Part model, mm, in its own coordinate system. Face numbers are marked on the shaded views. Give positions to 0.01 mm unless a question says otherwise; leave off trailing zeros. Write each loop counter-clockwise with the first axis right and the second up, starting at its lowest first coordinate (ties: lowest second). Pieces come first, ordered by that corner, then holes.
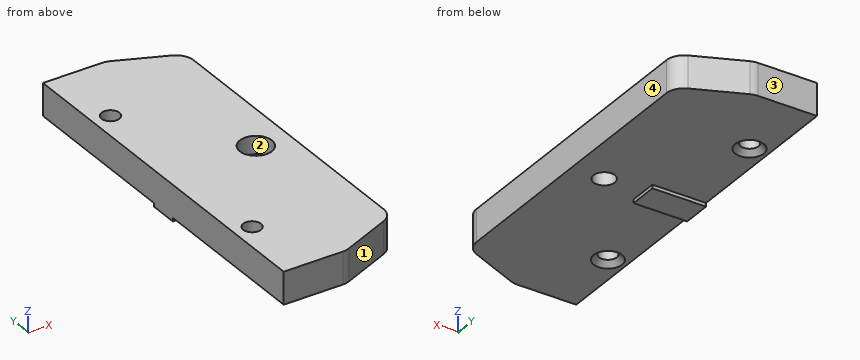
from build123d import *

# Parameters (mm, degrees)
F0_W           = 30
F0_H           = 16
F1_DEPTH       = 18
F2_D           = 12
F2_CBORE_D     = 18
F2_CBORE_DEPTH = 10
F3_DEPTH       = 20
F4_D           = 10
F4_CSINK_D     = 16
F4_CSINK_ANGLE = 90


with BuildPart() as f1:
    # F0 (on Top) → F1 (new body)
    with BuildSketch(Plane.XY):
        with BuildLine():
            Line((33.001347, 0), (0, 0))
            Line((0, 0), (0, -94))
            Line((0, -94), (30, -94))
            Line((30, -94), (30, -110))
            Line((30, -110), (0, -110))
            Line((0, -110), (0, -204))
            Line((0, -204), (33.001347, -204))
            ThreePointArc((33.001347, -204), (35.014898, -203.795183), (36.945967, -203.189123))
            Line((36.945967, -203.189123), (63.94462, -191.599396))
            ThreePointArc((63.94462, -191.599396), (68.350036, -187.912719), (70, -182.410274))
            Line((70, -182.410274), (70, -21.589726))
            ThreePointArc((70, -21.589726), (68.350036, -16.087281), (63.94462, -12.400604))
            Line((63.94462, -12.400604), (36.945967, -0.810877))
            ThreePointArc((36.945967, -0.810877), (35.014898, -0.204817), (33.001347, 0))
        make_face()
        with Locations((15, -102)):
            Rectangle(F0_W, F0_H)
    extrude(amount=-F1_DEPTH)

    # F2 (through all)
    with Locations(Plane.XY):
        with Locations((51.690422, -102)):
            CounterBoreHole(F2_D / 2, F2_CBORE_D / 2, F2_CBORE_DEPTH)

    # F0 (on Top) → F3 (join)
    with BuildSketch(Plane.XY):
        with Locations((15, -102)):
            Rectangle(F0_W, F0_H)
    extrude(amount=-F3_DEPTH)

    # F4 (through all)
    with Locations(Plane(origin=(0, 0, -18), x_dir=(1, 0, 0), z_dir=(0, 0, -1))):
        with Locations((10, 162), (10, 42)):
            CounterSinkHole(F4_D / 2, F4_CSINK_D / 2, counter_sink_angle=F4_CSINK_ANGLE)


solid = f1.part
1) Saw through at D-D (x = 21). Write the cut outline in (y, z), and give its area (3 significant figures).
Check result:
outline: (-204, -18) - (-110, -18) - (-110, -20) - (-94, -20) - (-94, -18) - (0, -18) - (0, 0) - (-204, 0) - close
area: 3,700 mm2
2) Drill centre lines: L1, parallel to Y at x = 10, z = -8.75; L2, parallel to X at y = -162, z = -10.75; L3, parallel to Z at x = 58, y = -124. Where is each one in solid material? Low to high.
Check result:
L1: y = -204 to -167, -157 to -47, -37 to 0
L2: x = 0 to 5, 15 to 70
L3: z = -18 to 0
3) Flat gauge pins, fed straight in: P1, Ø1, axis at x = 10, z = -19, coming from the -Y side; P2, Ø1, axis at y = -100, z = -19, coming from the +X side; P3, Ø6, axis at x = 10, y = -162, coming from the -Z side; P4, Ø2, axis at x = 10.5, z = -19.5, coming from the +Y side. Where does each tip first touch, or does it go through?
Check result:
P1: stops at y = -110
P2: stops at x = 30
P3: passes through
P4: stops at y = -94
4) Saw through at B-B (y = -102). Write the cut outline in (x, z), and give its area (3 significant figures).
Check result:
outline: (0, -20) - (30, -20) - (30, -18) - (45.69, -18) - (45.69, -10) - (42.69, -10) - (42.69, 0) - (0, 0) - close; (57.69, -18) - (70, -18) - (70, 0) - (60.69, 0) - (60.69, -10) - (57.69, -10) - close
area: 1,040 mm2
5) Saw through at C-C (z = -3.25). Write the cut outline in (x, y), and give its area (3 significant figures).
Check result:
outline: (0, -204) - (33, -204) arc R10 ccw to (36.95, -203.19) - (63.94, -191.6) arc R10 ccw to (70, -182.41) - (70, -21.59) arc R10 ccw to (63.94, -12.4) - (36.95, -0.81) arc R10 ccw to (33, 0) - (0, 0) - close; hole circle Ø10 at (10, -162); hole circle Ø10 at (10, -42); hole circle Ø18 at (51.69, -102)
area: 13,300 mm2
6) Saw through at A-A (x = 10). Write the cut outline in (y, z).
Check result:
outline: (-204, -18) - (-170, -18) - (-167, -15) - (-167, 0) - (-204, 0) - close; (-157, -15) - (-154, -18) - (-110, -18) - (-110, -20) - (-94, -20) - (-94, -18) - (-50, -18) - (-47, -15) - (-47, 0) - (-157, 0) - close; (-37, -15) - (-34, -18) - (0, -18) - (0, 0) - (-37, 0) - close
7) Mould opens along Y. For the marked faces 1, 2, 3 and 4 say: +Y half, -Y half, draft (parallel to the pull), parting line (faces both ways), or undercut.
Check result:
face 1: -Y half
face 2: undercut
face 3: +Y half
face 4: draft
